Geometry: see drawing. Coordinates: mm, zero at the bounding-box minimum. Give positions to 0.01 mm unless a question says otherwise; leave off trailing zeros. Loops run counter-clockwise (first coordinate to the right, second up) from the corner with the lowest first, then second, coordinate; pieces in that order, holes last. Notation, with made-up numbers: M -18.5,34.25 L -13.5,34.25 A30 cw -13.5,67.25 Z; hole C 14.5,85.25 d3. An arc over 180 degrees is marked long. Return JSON: item names as keys, results as strings. Group by question number.
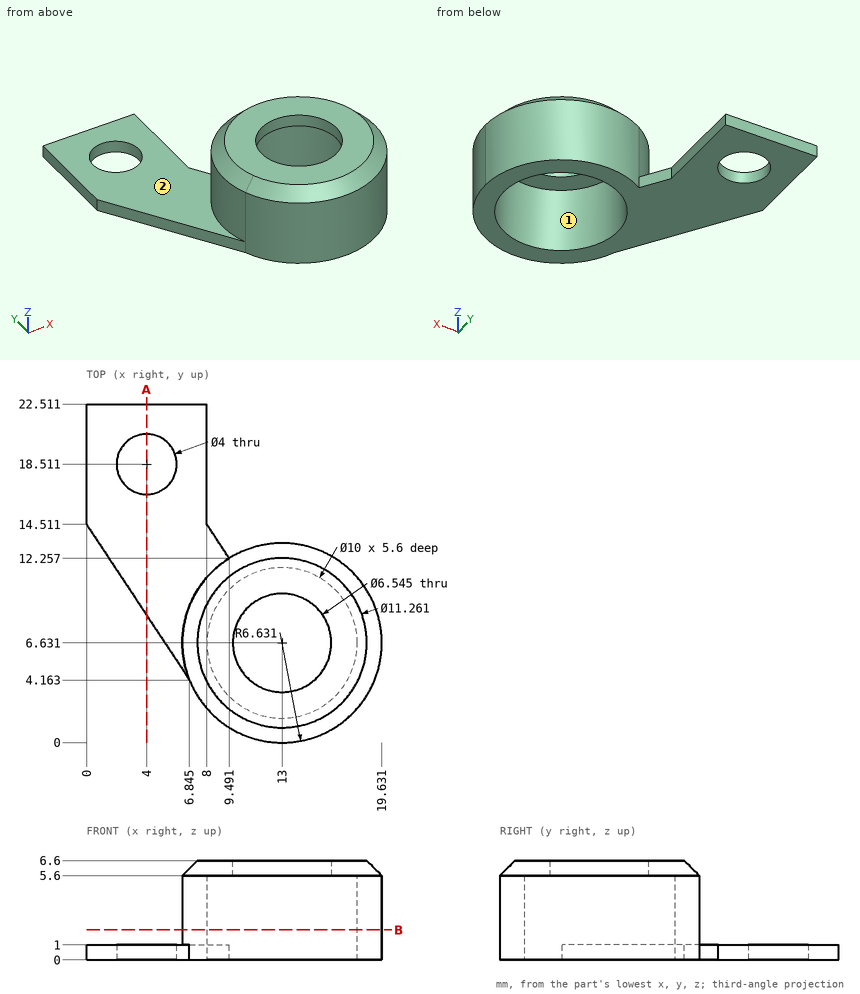
Item 1: First-contact query: pin 1 Ø8 at (x, y) = (13, 6.63) entering from -Z; pin 2 Ø3 at (x, y) = (4, 9.5) entering from +Z; pin 3 Ø0.5 at (y, z) = (19, 0.5) entering from +X. Flat tips, straight axial feed; report the tip coordinate or a pass-through.
Item 2: Section B-B, the plane z = 2. Return loops of the section in (x, y) (1 decimal).
Item 3: Material intervals for line 1 (X direction, y = 6.5, z = 2.75); line 2 (Z direction, x = 16.25, y = 4.25); line 3 (Y direction, x = 4, z = 0.2) (1 decimal), sorted ascending. Write a range as from..to.
Item 4: Section A-A, the plane x = 4. Return loops of the section in (y, z) (1 decimal).
Item 5: Pull-direction query (Y, two-part tool) for the marked faces 1 and 2; classes: pulls with the +Y half, pulls with the -Y half, needs draft (parallel to the pull), parting line crosses it, or undercut.
Answer below:
{
 "1": {"pin 1": "z = 5.6", "pin 2": "z = 1", "pin 3": "x = 8"},
 "2": {"outline": "M 6.8,4.2 A6.6 ccw 19.6,6.6 A6.6 ccw long Z; hole C 13,6.6 d10"},
 "3": {"line 1": "6.37..8, 18..19.63", "line 2": "5.6..6.6", "line 3": "8.5..16.5, 20.5..22.5"},
 "4": {"outline": "M 8.5,0 L 16.5,0 L 16.5,1 L 8.5,1 Z; M 20.5,0 L 22.5,0 L 22.5,1 L 20.5,1 Z"},
 "5": {"face 1": "undercut", "face 2": "needs draft"}
}
